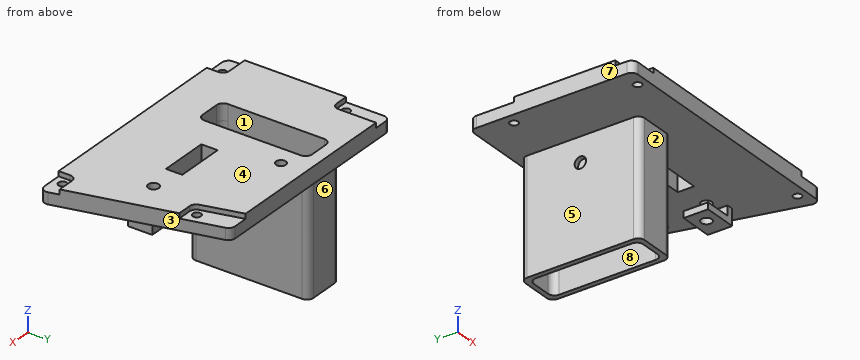
from build123d import *

# Parameters (mm, degrees)
BOSS_EXTRUDE1_DEPTH = 10
SKETCH2_R           = 3
SKETCH2_W           = 20
SKETCH2_H           = 67
SKETCH2_W_2         = 30
SKETCH2_H_2         = 10
CUT_EXTRUDE1_DEPTH  = 10
FILLET1_R           = 4
BOSS_EXTRUDE2_START = 70
BOSS_EXTRUDE2_DEPTH = 70
CUT_EXTRUDE5_DEPTH  = 3
SKETCH7_R           = 2.5
CUT_EXTRUDE6_DEPTH  = 7
CUT_EXTRUDE8_START  = -5
SKETCH8_R           = 3.5
CUT_EXTRUDE8_DEPTH  = 30
SKETCH9_W           = 4
SKETCH9_H           = 15
BOSS_EXTRUDE3_DEPTH = 10
SKETCH10_W          = 4
SKETCH10_H          = 15
BOSS_EXTRUDE4_DEPTH = 16.5
SKETCH5_R           = 3.25
CUT_EXTRUDE10_DEPTH = 20


with BuildPart() as part:
    # Sketch1 → Boss-Extrude1 (new body)
    with BuildSketch(Plane.XY):
        with BuildLine():
            Line((-38.056074766, 50.23364486), (89.820819608, 50.23364486))
            ThreePointArc((89.820819608, 50.23364486), (92.282468446, 49.386466612), (93.701389609, 47.20378736))
            Line((93.701389609, 47.20378736), (116.701389609, -44.79621264))
            ThreePointArc((116.701389609, -44.79621264), (115.97364136, -48.228003978), (112.820819608, -49.76635514))
            Line((112.820819608, -49.76635514), (-38.056074766, -49.76635514))
            ThreePointArc((-38.056074766, -49.76635514), (-40.884501891, -48.594782265), (-42.056074766, -45.76635514))
            Line((-42.056074766, -45.76635514), (-42.056074766, 46.23364486))
            ThreePointArc((-42.056074766, 46.23364486), (-40.884501891, 49.062071985), (-38.056074766, 50.23364486))
        make_face()
    extrude(amount=BOSS_EXTRUDE1_DEPTH)

    # Sketch2 → Cut-Extrude1 (cut)
    with BuildSketch(Plane.XY.offset(10)):
        with Locations((29.943925234, 35.23364486)):
            Circle(SKETCH2_R)
        with Locations((7.943925234, 9.23364486)):
            Rectangle(SKETCH2_W, SKETCH2_H)
        with Locations((52.943925234, -2.76635514)):
            Rectangle(SKETCH2_W_2, SKETCH2_H_2)
    extrude(amount=-CUT_EXTRUDE1_DEPTH, mode=Mode.SUBTRACT)

    # Fillet1
    fillet1_edges = [part.edges().sort_by_distance(p)[0] for p in [
        (-2.056074766, -24.26635514, 5),
        (-2.056074766, 42.73364486, 5),
        (17.943925234, 42.73364486, 5),
        (17.943925234, -24.26635514, 5),
    ]]
    fillet(fillet1_edges, radius=FILLET1_R)

    # Sketch4 → Boss-Extrude2 (add)
    with BuildSketch(Plane(origin=(0, 0, 0), x_dir=(-1, 0, 0), z_dir=(0, 0, -1)).offset(BOSS_EXTRUDE2_START)):
        with BuildLine():
            Line((-16.943925234, 45.73364486), (1.056074766, 45.73364486))
            ThreePointArc((1.056074766, 45.73364486), (3.884501891, 44.562071985), (5.056074766, 41.73364486))
            Line((5.056074766, 41.73364486), (5.056074766, -23.26635514))
            ThreePointArc((5.056074766, -23.26635514), (3.884501891, -26.094782265), (1.056074766, -27.26635514))
            Line((1.056074766, -27.26635514), (-16.943925234, -27.26635514))
            ThreePointArc((-16.943925234, -27.26635514), (-19.772352358, -26.094782265), (-20.943925234, -23.26635514))
            Line((-20.943925234, -23.26635514), (-20.943925234, 41.73364486))
            ThreePointArc((-20.943925234, 41.73364486), (-19.772352358, 44.562071985), (-16.943925234, 45.73364486))
        make_face()
        with BuildLine():
            Line((-1.943925234, -24.26635514), (-13.943925234, -24.26635514))
            ThreePointArc((-13.943925234, -24.26635514), (-16.772352358, -23.094782265), (-17.943925234, -20.26635514))
            Line((-17.943925234, -20.26635514), (-17.943925234, 38.73364486))
            ThreePointArc((-17.943925234, 38.73364486), (-16.772352358, 41.562071985), (-13.943925234, 42.73364486))
            Line((-13.943925234, 42.73364486), (-1.943925234, 42.73364486))
            ThreePointArc((-1.943925234, 42.73364486), (0.884501891, 41.562071985), (2.056074766, 38.73364486))
            Line((2.056074766, 38.73364486), (2.056074766, -20.26635514))
            ThreePointArc((2.056074766, -20.26635514), (0.884501891, -23.094782265), (-1.943925234, -24.26635514))
        make_face(mode=Mode.SUBTRACT)
    extrude(amount=-BOSS_EXTRUDE2_DEPTH)

    # Sketch6 → Cut-Extrude5 (cut)
    with BuildSketch(Plane.XY.offset(10)):
        with BuildLine():
            Line((-42.056074766, 50.23364486), (-30.056074766, 50.23364486))
            Line((-30.056074766, 50.23364486), (-30.056074766, 27.23364486))
            ThreePointArc((-30.056074766, 27.23364486), (-31.227647642, 24.405217735), (-34.056074766, 23.23364486))
            Line((-34.056074766, 23.23364486), (-42.056074766, 23.23364486))
            Line((-42.056074766, 23.23364486), (-42.056074766, 50.23364486))
        make_face()
        with BuildLine():
            Line((-25.056074766, -49.76635514), (-42.056074766, -49.76635514))
            Line((-42.056074766, -49.76635514), (-42.056074766, -38.76635514))
            Line((-42.056074766, -38.76635514), (-29.056074766, -38.76635514))
            ThreePointArc((-29.056074766, -38.76635514), (-26.227647642, -39.937928015), (-25.056074766, -42.76635514))
            Line((-25.056074766, -42.76635514), (-25.056074766, -49.76635514))
        make_face()
        with BuildLine():
            Line((80.820819608, 50.23364486), (87.044039625, 26.229796225))
            ThreePointArc((87.044039625, 26.229796225), (88.468109177, 24.070150388), (90.916027217, 23.23364486))
            Line((90.916027217, 23.23364486), (99.820819608, 23.23364486))
            Line((99.820819608, 23.23364486), (99.820819608, 50.23364486))
            Line((99.820819608, 50.23364486), (80.820819608, 50.23364486))
        make_face()
        with BuildLine():
            Line((100.820819608, -49.76635514), (116.820819608, -49.76635514))
            Line((116.820819608, -49.76635514), (116.820819608, -38.76635514))
            Line((116.820819608, -38.76635514), (104.820819608, -38.76635514))
            ThreePointArc((104.820819608, -38.76635514), (101.992392483, -39.937928015), (100.820819608, -42.76635514))
            Line((100.820819608, -42.76635514), (100.820819608, -49.76635514))
        make_face()
    extrude(amount=-CUT_EXTRUDE5_DEPTH, mode=Mode.SUBTRACT)

    # Sketch7 → Cut-Extrude6 (cut)
    with BuildSketch(Plane.XY.offset(7)):
        with Locations((91.68982912, 28.23364486)):
            Circle(SKETCH7_R)
        with Locations((-35.056074766, 28.23364486)):
            Circle(SKETCH7_R)
        with Locations((105.820819608, -43.76635514)):
            Circle(SKETCH7_R)
        with Locations((-30.056074766, -43.76635514)):
            Circle(SKETCH7_R)
    extrude(amount=-CUT_EXTRUDE6_DEPTH, mode=Mode.SUBTRACT)

    # Sketch8 → Cut-Extrude8 (cut)
    with BuildSketch(Plane(origin=(-1.056074766, 45.73364486, -70), x_dir=(0, 0, -1), z_dir=(1, 0, 0)).offset(CUT_EXTRUDE8_START)):
        with Locations(Location((-55, -36.5, 0), (0, 0, 270))):
            Circle(SKETCH8_R)
    extrude(amount=CUT_EXTRUDE8_DEPTH, mode=Mode.SUBTRACT)

    # Sketch9 → Boss-Extrude3 (add)
    with BuildSketch(Plane(origin=(0, 0, 0), x_dir=(-1, 0, 0), z_dir=(0, 0, -1))):
        with Locations((-94.943925234, -2.76635514)):
            Rectangle(SKETCH9_W, SKETCH9_H)
    extrude(amount=BOSS_EXTRUDE3_DEPTH)

    # Sketch10 → Boss-Extrude4 (add)
    with BuildSketch(Plane.ZY.offset(-92.943925234)):
        with Locations((-8, -2.76635514)):
            Rectangle(SKETCH10_W, SKETCH10_H)
    extrude(amount=BOSS_EXTRUDE4_DEPTH)

    # Sketch5 → Cut-Extrude10 (cut)
    with BuildSketch(Plane.XY.offset(10)):
        with Locations((85.443925234, -2.76635514)):
            Circle(SKETCH5_R)
    extrude(amount=-CUT_EXTRUDE10_DEPTH, mode=Mode.SUBTRACT)


solid = part.part
Can you work these out from the model? Positions are in its coordinate system, mm. Face numbers are marked on the shaded views. A direction names the side the tool comes from. Round coordinates to 2 decimals unless told otherwise and drop trailing zeros. Loops run counter-clockwise (first coordinate to the right, second up) from the corner with the lowest first, then second, coordinate; pieces in that order, holes last. Notation, with made-up numbers: (72.25, 80.25) - (78.25, 80.25) arc R21 cw to (78.25, 90.25) - close; hole circle Ø3 at (26, -28.75). An arc over 180 degrees is marked (long way). Answer in a Markdown table with one row per item. Add a question column.
Q1. I want a section at A-A on z = -15. List the corners of the cut face in (x, y) for me, and give its area (3 significant figures).
Q2. We'd pull the mould along Y, two halves only. Please class the marked faces 1, 2, 3 and 4: pulls with the +Y half, pulls with the -Y half, needs draft (parallel to the pull), parting line crosses it, or undercut.
Q3. Which directions (+Z, -Z, +X, -X, +Y, -Y) give clear straight access to the entire face, cutting with the end or side of a thin tool? Please do the marked faces 5, 6, 7 and 8.
Q4. For pin 1 Ø11 at (y, z) = (9.23, -15) entering from -X; pin 2 Ø1 at (x, y) = (-25.5, 4) entering from -Z; pin 3 Ø3 at (x, z) = (91.5, -3) entering from -Y, each with a flat end and sliding along its axis, tell me the tip position at first contact or that it passes through.
Q5. I want a section at C-C on z = -63.5. List the corners of the cut face in (x, y) for me, and give its area (3 significant figures).
Q6. I need wall thicknesses on L1, parallel to X at y = -17.5, z = -42; L2, parallel to Z at x = 81.5, y = 13; L3, parallel to Y at x = 92.5, z = -9. Which ranges of each line are inside material? Lowest first, please.
Q7. I want a section at B-B on y = 21. List the corners of the cut face in (x, z) for me, and give its area (3 significant figures).
Q8. I want a section at D-D on x = 106.5. List the corners of the cut face in (y, z) for me, and give its area (3 significant figures).
A:
| question | item | result |
|---|---|---|
| 1 | outline | (-5.06, -23.27) arc R4 ccw to (-1.06, -27.27) - (16.94, -27.27) arc R4 ccw to (20.94, -23.27) - (20.94, 5.73) - (17.94, 5.73) - (17.94, -20.27) arc R4 cw to (13.94, -24.27) - (1.94, -24.27) arc R4 cw to (-2.06, -20.27) - (-2.06, 5.73) - (-5.06, 5.73) - close; (-5.06, 12.73) - (-2.06, 12.73) - (-2.06, 38.73) arc R4 cw to (1.94, 42.73) - (13.94, 42.73) arc R4 cw to (17.94, 38.73) - (17.94, 12.73) - (20.94, 12.73) - (20.94, 41.73) arc R4 ccw to (16.94, 45.73) - (-1.06, 45.73) arc R4 ccw to (-5.06, 41.73) - close |
| 1 | area | 516 mm^2 |
| 2 | face 1 | undercut |
| 2 | face 2 | pulls with the -Y half |
| 2 | face 3 | pulls with the +Y half |
| 2 | face 4 | needs draft |
| 3 | face 5 | -Z, -X, +Y, -Y |
| 3 | face 6 | -Z, +X, -X, +Y |
| 3 | face 7 | +Z, -Z, -X, +Y, -Y |
| 3 | face 8 | +Z, -Z |
| 4 | pin 1 | x = -5.06 |
| 4 | pin 2 | z = 0 |
| 4 | pin 3 | y = -10.27 |
| 5 | outline | (-5.06, -23.27) arc R4 ccw to (-1.06, -27.27) - (16.94, -27.27) arc R4 ccw to (20.94, -23.27) - (20.94, 41.73) arc R4 ccw to (16.94, 45.73) - (-1.06, 45.73) arc R4 ccw to (-5.06, 41.73) - close; hole (-2.06, -20.27) arc R4 ccw to (1.94, -24.27) - (13.94, -24.27) arc R4 ccw to (17.94, -20.27) - (17.94, 38.73) arc R4 ccw to (13.94, 42.73) - (1.94, 42.73) arc R4 ccw to (-2.06, 38.73) - close |
| 5 | area | 558 mm^2 |
| 6 | L1 | -5.06 to -2.06, 17.94 to 20.94 |
| 6 | L2 | 0 to 10 |
| 6 | L3 | -10.27 to 4.73 |
| 7 | outline | (-42.06, 0) - (-5.06, 0) - (-5.06, -70) - (-2.06, -70) - (-2.06, 10) - (-42.06, 10) - close; (17.94, -70) - (20.94, -70) - (20.94, 0) - (100.25, 0) - (100.25, 10) - (17.94, 10) - close |
| 7 | area | 1,640 mm^2 |
| 8 | outline | (-49.77, 0) - (-46.17, 0) - (-46.17, 7) - (-49.77, 7) - close; (-41.36, 0) - (-3.99, 0) - (-3.99, 10) - (-38.77, 10) - (-38.77, 7) - (-41.36, 7) - close |
| 8 | area | 391 mm^2 |
